Part print with two shaded views. Sizes in mm from the minimum x, y, z corner. Round coordinates to 2 decimals unless told otherwise and drop trailing zeros. Order: outer loops, then holes, each group sorted by start corner. A loop starts at its lowest first (then second) coordinate and runs counter-clockwise, first axis right, second up. Notation, with made-up numbers: M 68,-37 L 114,-37 A30 cw 114,-4 Z; hole C -12.5,19.25 d6. An arc over 180 degrees is marked long. Put each result on its own line as item: value.
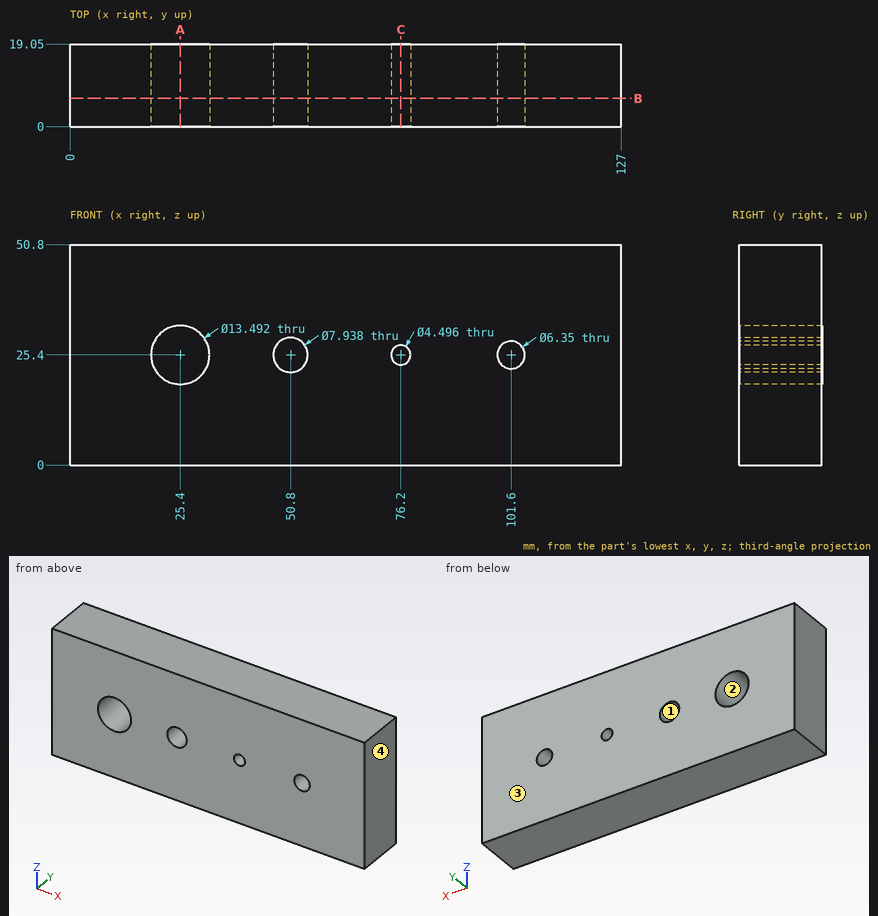
Item 1: Mould opens along X. For the marked faces 1, 2, 3 and 4 say: pulls with the +X half, pulls with the -X half, needs draft (parallel to the pull), parting line crosses it, or undercut.
Answers below:
face 1: undercut
face 2: undercut
face 3: needs draft
face 4: pulls with the +X half
Item 2: Band-saw the part on C-C on x = 76.2. Give the cut face in (y, z).
Answers below:
outline: M 0,0 L 19.05,0 L 19.05,23.15 L 0,23.15 Z; M 0,27.65 L 19.05,27.65 L 19.05,50.8 L 0,50.8 Z
Item 3: Probe line 1 along X through (y, z) = (10.25, 25.4) (1 decimal); line 2 along Z through (x, y) = (76.2, 12.75); line 3 along Z through (x, y) = (25.4, 12). List the from-to ranges inside material, lowest first. Write a range as [from, to].
Answers below:
line 1: [0, 18.7], [32.1, 46.8], [54.8, 74], [78.4, 98.4], [104.8, 127]
line 2: [0, 23.15], [27.65, 50.8]
line 3: [0, 18.65], [32.15, 50.8]
Item 4: Band-saw the part on A-A on x = 25.4. Give the cut face in (y, z).
Answers below:
outline: M 0,0 L 19.05,0 L 19.05,18.65 L 0,18.65 Z; M 0,32.15 L 19.05,32.15 L 19.05,50.8 L 0,50.8 Z
Item 5: Pin check, flat tip, straight feed: P1, Ø5.5, axis at x = 101.6, z = 25.4, coming from the -Y side. Stop position of the tip, or through.
Answers below:
P1: through
Item 6: Band-saw the part on B-B on y = 6.5. State how many separate pieces and enclosed holes the cut face has, and give its area (3 significant figures).
Answers below:
separate pieces: 1
enclosed holes: 4
area: 6,210 mm²
